Check sheet for the modelled part. Datum: model origin and axes. Units: mm. Face numbers are marked on the shaded views. A direction names the side the tool comes from. Coordinates: 2 decimals unless noted, no trailing zeros. Loops run counter-clockwise (first coordinate to the right, second up) from the corner with the lowest first, then second, coordinate; pieces in that order, holes last. Notation, with made-up numbers: (73.5, -2) -> (84.5, -2) arc R29 cw to (84.5, 26) -> close; hole circle Ø10 at (13, -4). An arc over 180 degrees is marked (long way). Use CSV: the item, a comma, the result in double quotes. Start each with the question number.
1. Set-up check for the marked faces 5, 6 and 7: record each of +Z, -Z, +X, -X, +Y, -Y from which the full face is reachable in a straight line by a thin tool's end or side.
2. Sectioned sample at D-D, the plane x = 85. Record the cut outline in (y, z), and give its area (3 significant figures).
3. Sectioned sample at C-C, the plane z = 1046. Record the cut outline in (x, y), and give its area (3 significant figures).
4. Thickness scan on L1, parallel to X at y = -159.5, z = 631; L2, parallel to X at y = -177.5, z = 999; L3, parallel to X at y = -57, z = 1250. Record the ranges inside material, lowest first.
5. Release check for a two-part mould opening along X. For the marked faces 1, 2, 3 and 4 record: pulls with the +X half, pulls with the -X half, needs draft (parallel to the pull), parting line crosses it, or undercut.
6. Gauge pin test, flat ends, axial feed: pin 1 (6 mm diameter, centred on x = 727.5, z = 943, fed in from +Y); pin 2 (8 mm diameter, centred on x = 769, z = 863.5, fed in from -Y); pin 3 (1 mm diameter, centred on x = 748, y = -110, fed in from -Z). Record the tip position at first contact, or that the pin passes through.
7. Sectioned sample at B-B, the plane x = 333.5. Record the cut outline in (y, z).
8. Sectioned sample at A-A, the plane y = -242. Record the cut outline in (x, z).
```python
from build123d import *

# Parameters (mm, degrees)
F0_W     = 914.4
F0_H     = 1371.6
F1_DEPTH = 304.8
F2_W     = 571.5
F2_H     = 1130.3
F2_W_2   = 279.4
F2_H_2   = 990.6
F2_H_3   = 203.2
F3_DEPTH = 279.4


with BuildPart() as f1:
    # F0 (on Front) → F1 (new body)
    with BuildSketch(Plane.XZ):
        with Locations((457.2, 685.8)):
            Rectangle(F0_W, F0_H)
    extrude(amount=F1_DEPTH)

    # F2 (on face) → F3 (cut, through all)
    with BuildSketch(Plane.XZ.offset(304.8)):
        with Locations((603.25, 565.15)):
            Rectangle(F2_W, F2_H)
        with Locations((165.1, 495.3)):
            Rectangle(F2_W_2, F2_H_2)
        with Locations((165.1, 1244.6)):
            Rectangle(F2_W_2, F2_H_3)
        with Locations((457.2, 1244.6)):
            Rectangle(F2_W_2, F2_H_3)
        with Locations((749.3, 1244.6)):
            Rectangle(F2_W_2, F2_H_3)
    extrude(amount=-F3_DEPTH, mode=Mode.SUBTRACT)


solid = f1.part
```
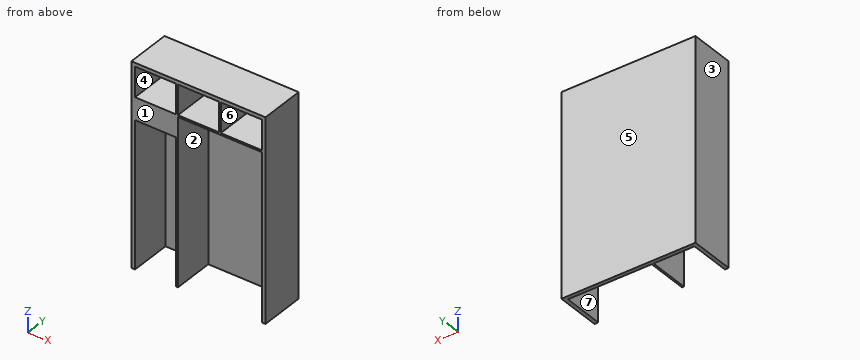
Completed:
1,face 5,"+Z, -Z, +X, -X, +Y"
1,face 6,"-Y"
1,face 7,"-Z, -Y"
2,outline,"(-304.8, 990.6) -> (-25.4, 990.6) -> (-25.4, 0) -> (0, 0) -> (0, 1371.6) -> (-304.8, 1371.6) -> (-304.8, 1346.2) -> (-25.4, 1346.2) -> (-25.4, 1143) -> (-304.8, 1143) -> close"
2,area,"84,500 mm²"
3,outline,"(0, -304.8) -> (317.5, -304.8) -> (317.5, -25.4) -> (889, -25.4) -> (889, -304.8) -> (914.4, -304.8) -> (914.4, 0) -> (0, 0) -> close"
3,area,"119,000 mm²"
4,L1,"0 to 25.4, 304.8 to 317.5, 889 to 914.4"
4,L2,"0 to 317.5, 889 to 914.4"
4,L3,"0 to 25.4, 304.8 to 317.5, 596.9 to 609.6, 889 to 914.4"
5,face 1,"needs draft"
5,face 2,"undercut"
5,face 3,"pulls with the -X half"
5,face 4,"undercut"
6,pin 1,"y = 0"
6,pin 2,"y = -25.4"
6,pin 3,"z = 1130.3"
7,outline,"(-304.8, 1130.3) -> (-25.4, 1130.3) -> (-25.4, 0) -> (0, 0) -> (0, 1371.6) -> (-304.8, 1371.6) -> (-304.8, 1346.2) -> (-25.4, 1346.2) -> (-25.4, 1143) -> (-304.8, 1143) -> close"
8,outline,"(0, 0) -> (25.4, 0) -> (25.4, 990.6) -> (304.8, 990.6) -> (304.8, 0) -> (317.5, 0) -> (317.5, 1130.3) -> (889, 1130.3) -> (889, 0) -> (914.4, 0) -> (914.4, 1371.6) -> (0, 1371.6) -> close; hole (25.4, 1143) -> (304.8, 1143) -> (304.8, 1346.2) -> (25.4, 1346.2) -> close; hole (317.5, 1143) -> (596.9, 1143) -> (596.9, 1346.2) -> (317.5, 1346.2) -> close; hole (609.6, 1143) -> (889, 1143) -> (889, 1346.2) -> (609.6, 1346.2) -> close"
